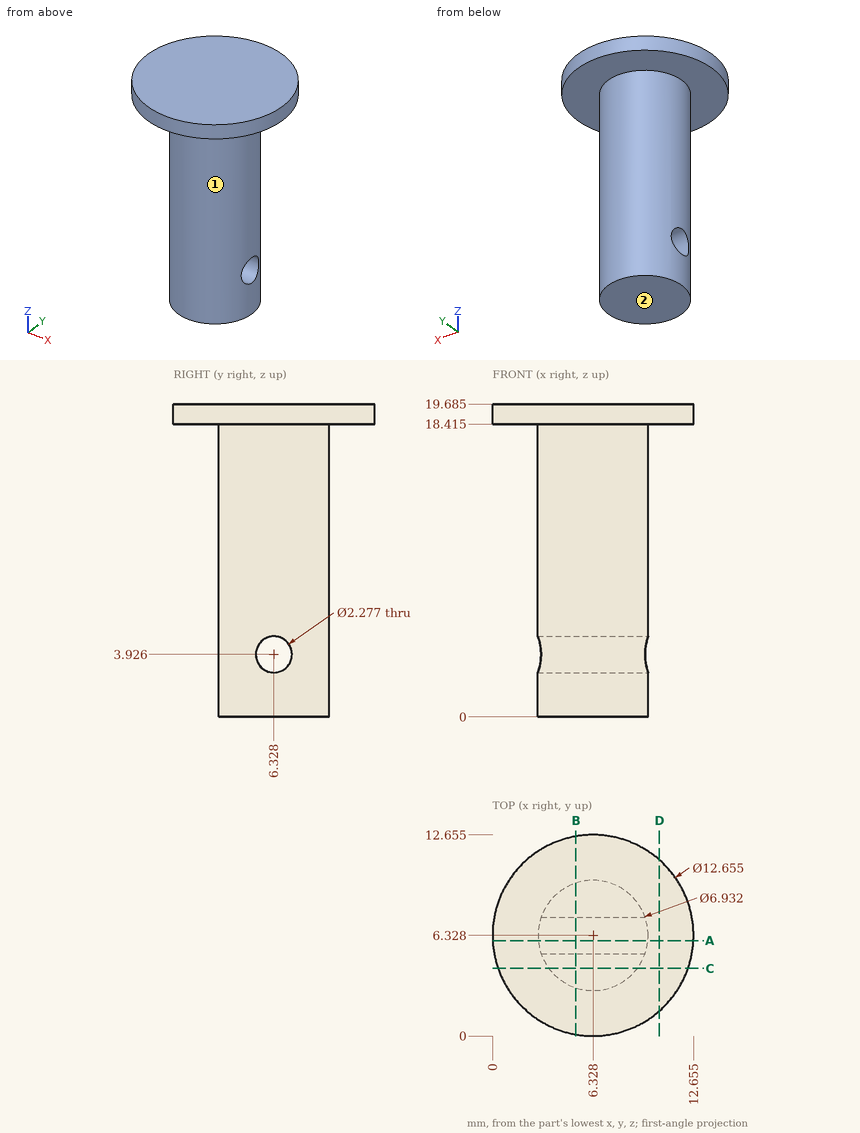
Part print with two shaded views. Sizes in mm from the minimum x, y, z corner. A direction names the side the tool comes from. Coordinates: 2 decimals unless noted, no trailing zeros. Write each loop counter-clockwise with the first axis right and the second up, starting at its lowest first coordinate (ties: lowest second). Pieces come first, ordered by that corner, then holes.
(1) Drill centre lines: line 1 (X direction, y = 6.25, z = 13.75); line 2 (Y direction, x = 6.5, z = 18.75); line 3 (Z direction, x = 5, y = 11) (1 decimal). Where is each one in solid material? Low to high.
(2) Cut at C-C on y = 4.25. List the corners of the cut face in (x, z) (1 decimal).
(3) Cut at B-B on x = 5.25. List the corners of the cut face in (y, z) (1 decimal).
(4) 3-axis set-ups, long thin cutter, end or side, ignore diameter. For the marked faces 1 and 2: which of +Z, -Z, +X, -X, +Y, -Y reach the whole face in a straight line?
(5) Cut at D-D on x = 10.5. List the corners of the cut face in (y, z) (1 decimal).
(6) Pin check, flat tips, straight feed: pin 1 Ø1 at (x, z) = (11, 14.5) entering from -Y; pin 2 Ø6 at (y, z) = (8, 14) entering from -X; pin 3 Ø2 at (y, z) = (4.5, 14) entering from -X; pin 4 Ø5 at (y, z) = (9.5, 3.5) entering from +X. Stop position of each tip, or through.
(7) Cut at A-A on y = 6. List the corners of the cut face in (x, z) (1 decimal), and give its area (3 significant figures).
Working result:
1. line 1: x = 2.86 to 9.79
1. line 2: y = 0 to 12.65
1. line 3: z = 18.4 to 19.7
2. outline: (0.4, 18.4) - (3.6, 18.4) - (3.6, 0) - (9.1, 0) - (9.1, 18.4) - (12.3, 18.4) - (12.3, 19.7) - (0.4, 19.7) - close
3. outline: (0.1, 18.4) - (3, 18.4) - (3, 0) - (9.6, 0) - (9.6, 18.4) - (12.6, 18.4) - (12.6, 19.7) - (0.1, 19.7) - close; hole circle Ø2.3 at (6.3, 3.9)
4. face 1: -Z
4. face 2: -Z, +X, -X, +Y, -Y
5. outline: (1.6, 18.4) - (11.1, 18.4) - (11.1, 19.7) - (1.6, 19.7) - close
6. pin 1: passes through
6. pin 2: stops at x = 2.86
6. pin 3: stops at x = 2.96
6. pin 4: stops at x = 9.72
7. outline: (0, 18.4) - (2.9, 18.4) - (2.9, 5) - (9.8, 5) - (9.8, 18.4) - (12.6, 18.4) - (12.6, 19.7) - (0, 19.7) - close; (2.9, 0) - (9.8, 0) - (9.8, 2.8) - (2.9, 2.8) - close
7. area: 128 mm2
